Check sheet for the modelled part. Datum: model origin and axes. Units: mm. A direction names the side the tool comes from. Round coordinates to 2 decimals unless told otherwise and drop trailing zeros. Write each loop counter-clockwise with the first axis right and the second up, starting at its lowest first coordinate (ties: lowest second). Pieces come first, ordered by that corner, then holes. Notation, with made-up numbers: (52.5, 54.25) -> (109.5, 54.25) arc R8 cw to (109.5, 63.25) -> close; hole circle Ø4 at (32, -32). An arc over 180 degrees is marked (long way). One line per item, written item: value.
Autodesk Inventor part; units mm, degrees
ref_plane "YZ Plane" through (0, 0, 0) normal (1, 0, 0) x (0, 1, 0)
ref_plane "XZ Plane" through (0, 0, 0) normal (0, 1, 0) x (-1, 0, 0)
ref_plane "XY Plane" through (0, 0, 0) normal (0, 0, 1) x (1, 0, 0)
sketch "Sketch1" plane through (0, 0, 0) normal (0, 0, 1) x (1, 0, 0)
  line L0 (-25, -40) -> (25, -40)
  line L1 (25, -40) -> (25, 40)
  line L2 (25, 40) -> (-25, 40)
  line L3 (-25, 40) -> (-25, -40)
  line L4 (-25, -40) -> (25, 40) construction
  line L5 (25, -40) -> (-25, 40) construction
  point P0 (0, 0)
  dimension "d0" = 50
  dimension "d1" = 80
extrude "Extrusion1" add sketch "Sketch1" along normal blind 6
sketch "Sketch2" plane through (-25, -40, 0) normal (0, -1, 0) x (1, 0, 0)
  line L0 (0, 6) -> (50, 6)
  line L1 (12, 6) -> (18, 6)
  line L2 (18, 6) -> (18, 3)
  line L3 (18, 3) -> (12, 3)
  line L4 (12, 3) -> (12, 6)
  line L5 (32, 6) -> (38, 6)
  line L6 (38, 6) -> (38, 3)
  line L7 (38, 3) -> (32, 3)
  line L8 (32, 3) -> (32, 6)
  line L9 (25, -1.2) -> (25, 7.2) construction
  line L10 (0, 0) -> (50, 0) construction
  line L11 (50, 0) -> (50, 6) construction
  line L12 (0, 6) -> (50, 6) construction
  line L13 (0, 0) -> (0, 6) construction
  point P0 (25, 0)
  point P1 (32, 4.5)
  point P2 (18, 4.5)
  dimension "d4" = 14
  dimension "d5" = 6
  dimension "d7" = 3
extrude "Extrusion2" cut sketch "Sketch2" against normal through all
fillet "Fillet1" radius 5 4 edges at (-25, 40, 3) (-25, -40, 3) (25, -40, 3) (25, 40, 3)
properties part number "Plate" material "Steel"
Item 1: Release check for a two-part mould opening along X. For faces 1 (the cylindrical face through (24, 38, 3)), 2 (the flat face through (-19, 1, 6)), 3 (the flat face through (-7, -1, 5)) record: pulls with the +X half, pulls with the -X half, needs draft (parallel to the pull), parting line crosses it, or undercut.
Result set:
face 1: pulls with the +X half
face 2: needs draft
face 3: undercut
Item 2: Sectioned sample at B-B (y = -4.5). Enter the section's corners in (x, z).
Result set:
outline: (-25, 0) -> (25, 0) -> (25, 6) -> (13, 6) -> (13, 3) -> (7, 3) -> (7, 6) -> (-7, 6) -> (-7, 3) -> (-13, 3) -> (-13, 6) -> (-25, 6) -> close
Item 3: Tool access check on faces 4 (the flat face through (-25, 0, 3)), 5 (the flat face through (7, -1, 4)). Record the directions out of +Z, -Z, +X, -X, +Y, -Y that give a thin tool (end or side, any length) a straight path to the whole face; none if there is none.
Result set:
face 4: +Z, -Z, -X, +Y, -Y
face 5: +Z, +Y, -Y
Item 4: Sectioned sample at A-A (z = 5). Enter the section's corners in (x, y), then the cut area to 3 significant figures.
Result set:
outline: (-25, -35) arc R5 ccw to (-20, -40) -> (-13, -40) -> (-13, 40) -> (-20, 40) arc R5 ccw to (-25, 35) -> close; (-7, -40) -> (7, -40) -> (7, 40) -> (-7, 40) -> close; (13, -40) -> (20, -40) arc R5 ccw to (25, -35) -> (25, 35) arc R5 ccw to (20, 40) -> (13, 40) -> close
area: 3,020 mm^2
Item 5: Depth check by flat-ended pin: pin 1 (1.8 mm diameter, centred on x = -11.5, y = 14, fed in from +Z). Enter the tip coordinate at first touch or a pass-through.
Result set:
pin 1: z = 3
Item 6: Material ranges on line 1 along X through (y, z) = (-11.5, 3.05); line 2 along Z through (x, y) = (-8.5, 19); line 3 along Y through (x, z) = (21.5, 5.7), recorded low to high.
Result set:
line 1: -25 to -13, -7 to 7, 13 to 25
line 2: 0 to 3
line 3: -39.77 to 39.77
